The listing builds one solid part. Answer for the finished solid, in the listing's coordinates (mm). Give positions to 0.01 mm unless a question says otherwise; leave off trailing zeros. Write each loop counter-clockwise with the first axis right and the second up, starting at its lowest first coordinate (ties: lowest second). Pieces come first, ordered by that corner, then holes. Notation, with made-up numbers: M 86.25,66 L 127.25,66 A21 cw 127.25,76 Z; hole C -17.75,22.25 d3. An arc over 180 degrees is marked long. Answer as a JSON object with one key per item and string values.
```python
from build123d import *

# Parameters (mm, degrees)
SALIENTE_EXTRUIR1_DEPTH = 0.1


with BuildPart() as part:
    # Model → Saliente-Extruir1 (new body)
    with BuildSketch(Plane.XY):
        with BuildLine():
            Line((14.734818135, -5.091278375), (14.734818135, -1.303795454))
            Line((14.734818135, -1.303795454), (9.586125983, 24.133225595))
            ThreePointArc((9.586125983, 24.133225595), (5.468112004, 27.581522666), (0.631193944, 25.246353401))
            ThreePointArc((0.631193944, 25.246353401), (-0.474240962, 16.497831322), (-0.079037247, 7.688606673))
            ThreePointArc((-0.079037247, 7.688606673), (-1.286055473, 1.941103292), (-1.312470922, -3.931714629))
            ThreePointArc((-1.312470922, -3.931714629), (2.054115678, -5.399292803), (5.726611642, -5.420843381))
            ThreePointArc((5.726611642, -5.420843381), (6.52637867, 0.347218865), (6.371178308, 6.168394193))
            ThreePointArc((6.371178308, 6.168394193), (8.138725842, 10.560479173), (9.052593122, 15.205851208))
            ThreePointArc((9.052593122, 15.205851208), (9.320849308, 4.901113732), (11.037087709, -5.263240729))
            Line((11.037087709, -5.263240729), (14.734818135, -5.091278375))
        make_face()
    extrude(amount=SALIENTE_EXTRUIR1_DEPTH)


solid = part.part
```
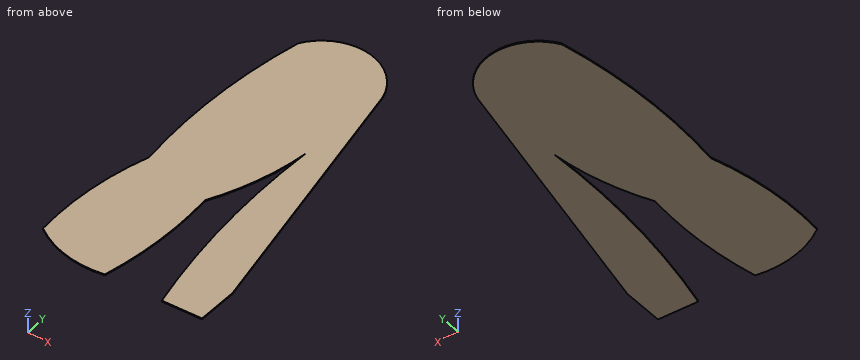
1. Consider line 1 along X through (y, z) = (3.5, 0.05); line 2 along X through (y, z) = (6, 0.05); line 3 along Y through (x, z) = (2.5, 0.05). Determine where each line is inside the solid, lowest interval first.
Verdict:
{"line 1": "x = -1.08 to 6.56, 9.47 to 13.76", "line 2": "x = -0.56 to 6.39, 9.22 to 13.26", "line 3": "y = -5.48 to 27.02"}
2. A cutting plane is placed at C-C, the plane y = -1. Give the vertices of the cut face in (x, z).
Verdict:
{"outline": "M -1.45,0 L 6.43,0 L 6.43,0.1 L -1.45,0.1 Z; M 10.14,0 L 14.67,0 L 14.67,0.1 L 10.14,0.1 Z"}
3. A flat-ended cylindrical pin translates along its axis: pin 1 (4 mm diameter, centred on x = 11, y = 17.5, fed in from -Z). Find the tip coordinate at first contact, or state that the pin passes through.
Verdict:
{"pin 1": "stops at z = 0"}
4. A cutting plane is placed at B-B, the plane y = 6.5. Give the vertices of the cut face in (x, z).
Verdict:
{"outline": "M -0.43,0 L 6.54,0 L 6.54,0.1 L -0.43,0.1 Z; M 9.18,0 L 13.16,0 L 13.16,0.1 L 9.18,0.1 Z"}
5. A cutting plane is placed at A-A, the plane z = 0.05. Give the vertices of the cut face in (x, y).
Verdict:
{"outline": "M -1.31,-3.93 A9.13 ccw 5.73,-5.42 A35.45 ccw 6.37,6.17 A25.17 ccw 9.05,15.21 A73.04 ccw 11.04,-5.26 L 14.73,-5.09 L 14.73,-1.3 L 9.59,24.13 A4.95 ccw 0.63,25.25 A51.77 ccw -0.08,7.69 A29.05 ccw Z"}
6. A cutting plane is placed at D-D, the plane x = 11.5. Give the vertices of the cut face in (y, z).
Verdict:
{"outline": "M -5.24,0 L 14.68,0 L 14.68,0.1 L -5.24,0.1 Z"}
